Geometry: final body of the model. Coordinates: model frame, mm. A direction names the side the tool comes from. Give positions to 0.01 mm unless a question says otherwise; leave off trailing zeros. Write each loop counter-clockwise with the first axis right and the second up, starting at its lowest first coordinate (ties: lowest second). Pieces come first, ordered by that corner, then holes. Notation, with made-up numbers: (-13.5, 21.25) -> (40.5, 21.25) arc R27 cw to (40.5, 47.25) -> close; hole circle Ø3 at (49, 62.5). An arc over 180 degrees is marked (long way). Answer as a JSON object with one key per item and string values.
from build123d import *

# Parameters (mm, degrees)
F0_R     = 10
F0_R_2   = 5.25
F1_DEPTH = 10
F2_R     = 5.25
F2_R_2   = 2.25
F3_DEPTH = 3
F4_SIZE  = 2
F5_SIZE2 = 2
F5_SIZE  = 8


with BuildPart() as f1:
    # F0 (on Top) → F1 (new body)
    with BuildSketch(Plane.XY):
        Circle(F0_R)
        Circle(F0_R_2, mode=Mode.SUBTRACT)
    extrude(amount=F1_DEPTH)

    # F2 (on Top) → F3 (join)
    with BuildSketch(Plane.XY):
        Circle(F2_R)
        Circle(F2_R_2, mode=Mode.SUBTRACT)
    extrude(amount=F3_DEPTH)

    # F4
    f4_edges = [f1.edges().sort_by_distance(p)[0] for p in [
        (-2.25, 0, 0),
    ]]
    chamfer(f4_edges, length=F4_SIZE)

    # F5
    f5_edges = [f1.edges().sort_by_distance(p)[0] for p in [
        (-10, 0, 0),
    ]]
    f5_side = f1.faces().sort_by_distance((-10, 0, 5))[0]
    chamfer(f5_edges, length=F5_SIZE, length2=F5_SIZE2, reference=f5_side)


solid = f1.part
Q1. Cut plane C-C (z = 5). Return the cut outline in (x, y), and give its area (3 significant figures).
Values:
{"outline": "circle Ø18.5 at (0, 0); hole circle Ø10.5 at (0, 0)", "area": "182 mm²"}
Q2. Set-up query: faces 1 (the cylindrical face through (5, 1.6, 6.5)), 2 (the cylindrical face through (-0.29, 2.23, 2.49)). Return all of +Z, -Z, +X, -X, +Y, -Y with unobstructed straight access to the full face (end or side cutting, diameter ignored); none if empty.
Values:
{"face 1": "+Z", "face 2": "+Z, -Z"}
Q3. Cut plane D-D (z = 8.75). Return the cut outline in (x, y), and give its area (3 significant figures).
Values:
{"outline": "circle Ø20 at (0, 0); hole circle Ø10.5 at (0, 0)", "area": "228 mm²"}
Q4. Material intervals for L1, parallel to Y at x = 0, z = 2.2; L2, parallel to X at y = 3, z = 7.25; L3, parallel to X at y = 4.25, z = 4.75, sorted ascending. Write a range as from..to.
Values:
{"L1": "-8.55..-2.25, 2.25..8.55", "L2": "-9.34..-4.31, 4.31..9.34", "L3": "-8.15..-3.08, 3.08..8.15"}
Q5. First-contact query: P1, Ø5, axis at x = 4, z = 7.5, coming from the -Y side; P2, Ø1, axis at x = -5.5, z = 7, coming from the +Y side; P3, Ø3, axis at x = -1.5, y = 2, coming from the +Z side. Flat tips, straight axial feed; report the tip coordinate or a pass-through.
Values:
{"P1": "y = -9.88", "P2": "y = 8.4", "P3": "z = 3"}
Q6. Mould query, pull axis Y, two halves, no side actions, for faces 3 (the flat face through (3.4, -3.4, 0)), 4 (the flat face through (2.3, -1.1, 3)), 5 (the cylindrical face through (-2.17, -9.76, 8.99)), 6 (the conical face through (2.27, 0.71, 1.87)). Classes: pulls with the +Y half, pulls with the -Y half, needs draft (parallel to the pull), parting line crosses it, or undercut.
Values:
{"face 3": "needs draft", "face 4": "undercut", "face 5": "parting line crosses it", "face 6": "undercut"}
Q7. Cut plane A-A (x = 0). Return the cut outline in (y, z), and give its area (3 significant figures).
Values:
{"outline": "(-10, 8) -> (-8, 0) -> (-4.25, 0) -> (-2.25, 2) -> (-2.25, 3) -> (-5.25, 3) -> (-5.25, 10) -> (-10, 10) -> close; (2.25, 2) -> (4.25, 0) -> (8, 0) -> (10, 8) -> (10, 10) -> (5.25, 10) -> (5.25, 3) -> (2.25, 3) -> close", "area": "93.0 mm²"}
